Could you check a few things on this model? Use its own coordinates, in mm. A direction names the side the tool comes from. Coordinates: 2 decimals unless noted, no trailing zeros. Loops run counter-clockwise (first coordinate to the right, second up) from the corner with the lowest first, then second, coordinate; pieces in that order, holes last. Notation, with made-up numbers: (-38, 57) -> (-6, 57) arc R23 ccw to (-6, 88) -> close; hole circle Ø5 at (2.25, -6.75). An arc over 180 degrees is marked (long way). One line per question, with ' | ' between items.
```python
from build123d import *

# Parameters (mm, degrees)
SKETCH001_R       = 23.34615
EXTRUDE_DEPTH     = 23
CYLINDER002_R     = 3
CYLINDER002_DEPTH = 15
CYLINDER001_R     = 7.5
CYLINDER001_DEPTH = 1
CYLINDER_R        = 11.5
CYLINDER_DEPTH    = 40
SKETCH_R          = 1
POCKET_DEPTH      = 4


with BuildPart() as clone_of_extrude:
    # Sketch001 → Extrude (new body)
    with BuildSketch(Plane.XY.offset(41)):
        Circle(SKETCH001_R)
    extrude(amount=EXTRUDE_DEPTH)


with BuildPart() as cylinder002:
    # Cylinder002 → Cylinder002 (new body)
    with BuildSketch(Plane.XY.offset(42)):
        Circle(CYLINDER002_R)
    extrude(amount=CYLINDER002_DEPTH)


with BuildPart() as cylinder001:
    # Cylinder001 → Cylinder001 (new body)
    with BuildSketch(Plane.XY.offset(41)):
        Circle(CYLINDER001_R)
    extrude(amount=CYLINDER001_DEPTH)


with BuildPart() as cut:
    # Cylinder → Cylinder (new body)
    with BuildSketch(Plane.XY.offset(1)):
        Circle(CYLINDER_R)
    extrude(amount=CYLINDER_DEPTH)

    # Fusion: union Cylinder002, Cylinder001
    add(cylinder002.part)
    add(cylinder001.part)

    # Sketch → Pocket (cut)
    with BuildSketch(Plane.XY.offset(41)):
        with Locations((8.227241, 4.75)):
            Circle(SKETCH_R)
        with Locations((-8.227241, 4.75)):
            Circle(SKETCH_R)
        with Locations((0, -9.5)):
            Circle(SKETCH_R)
    extrude(amount=-POCKET_DEPTH, mode=Mode.SUBTRACT)

    # Cut: cut Clone of Extrude
    add(clone_of_extrude.part, mode=Mode.SUBTRACT)


solid = cut.part
```
Q1. Imagine slicing it at B-B on z = 23.5. Write out the boundary of the cut face in (x, y).
Values follow:
outline: circle Ø23 at (0, 0)
Q2. For faces 5 (the face through (0, 0, 41)), 6 (the face through (9.18, 5.05, 39.03)), which set-ups out of +Z, -Z, +X, -X, +Y, -Y let a thin tool reach every point of the face, with its end or its side?
Values follow:
face 5: +Z, +X, -X, +Y, -Y | face 6: +Z
Q3. Please list where these lines run through material, in increasing order: L1, parallel to Y at x = 0, z = 39.3; L2, parallel to Y at x = -7.25, z = 36; L3, parallel to Y at x = 1.5, z = 9. Write a range as [from, to].
Values follow:
L1: y = [-11.5, -10.5], [-8.5, 11.5] | L2: y = [-8.93, 8.93] | L3: y = [-11.4, 11.4]
Q4. Imagine slicing it at C-C on x = 5.5. Write out the boundary of the cut face in (y, z).
Values follow:
outline: (-10.1, 1) -> (10.1, 1) -> (10.1, 41) -> (-10.1, 41) -> close
Q5. For pin 1 (1 mm diameter, centred on x = 6, z = 18, fed in from +Y); pin 2 (8 mm diameter, centred on y = -9, z = 20, fed in from -X); pin 3 (1.5 mm diameter, centred on y = 3, z = 16.5, fed in from +X), each with a flat end and sliding along its axis, tell me the tip position at first contact or that it passes through.
Values follow:
pin 1: stops at y = 10.1 | pin 2: stops at x = -10.36 | pin 3: stops at x = 11.28
Q6. We'd pull the mould along Y, two halves only. Please class faces 1 (the face through (-8, 5, 37)), 2 (the face through (-1.5, 11.4, 20.7)), 3 (the face through (0, -9, 37)), 4 (the face through (0, 0, 1)): released by +Y, released by -Y, zero draft, split by the parting line, or undercut.
Values follow:
face 1: undercut | face 2: split by the parting line | face 3: undercut | face 4: zero draft
Q7. Imagine slicing it at D-D on y = -9.5. Write out the boundary of the cut face in (x, z), plus the area to 3 significant figures.
Values follow:
outline: (-6.48, 1) -> (6.48, 1) -> (6.48, 41) -> (1, 41) -> (1, 37) -> (-1, 37) -> (-1, 41) -> (-6.48, 41) -> close | area: 510 mm2
Q8. Imagine slicing it at A-A on y = 4.75. Write out the boundary of the cut face in (x, z), plus the area to 3 significant figures.
Values follow:
outline: (-10.47, 1) -> (10.47, 1) -> (10.47, 41) -> (9.23, 41) -> (9.23, 37) -> (7.23, 37) -> (7.23, 41) -> (-7.23, 41) -> (-7.23, 37) -> (-9.23, 37) -> (-9.23, 41) -> (-10.47, 41) -> close | area: 822 mm2
